The listing builds one solid part. Answer for the finished solid, in the listing's coordinates (mm). Give positions to 0.01 mm unless a question says otherwise; leave off trailing zeros. Write each loop counter-clockwise with the first axis right and the second up, starting at its lowest first coordinate (ties: lowest second). Pieces come first, ordered by that corner, then holes.
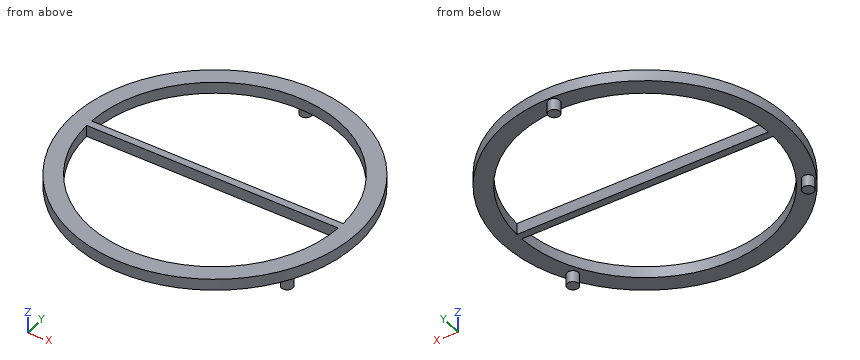
Autodesk Inventor part; units mm, degrees
ref_plane "YZ Plane" through (0, 0, 0) normal (1, 0, 0) x (0, 1, 0)
ref_plane "XZ Plane" through (0, 0, 0) normal (0, 1, 0) x (-1, 0, 0)
ref_plane "XY Plane" through (0, 0, 0) normal (0, 0, 1) x (1, 0, 0)
sketch "Sketch1" plane through (0, 0, 0) normal (0, 0, 1) x (1, 0, 0)
  circle A0 centre (0, 0) radius 250
  circle A1 centre (0, 0) radius 220
  dimension "d0" = 500
  dimension "d1" = 30
extrude "Extrusion1" add sketch "Sketch1" along normal blind 20
sketch "Sketch2" plane through (0, 0, 0) normal (0, 0, -1) x (-1, 0, 0)
  circle A0 centre (0, 237.6296) radius 10
  circle A1 centre (-205.7933, -118.8148) radius 10
  circle A2 centre (205.7933, -118.8148) radius 10
  point P0 (0, 0)
  dimension "d4" = 20
  dimension "d7" = 360
extrude "Extrusion2" add sketch "Sketch2" along normal blind 20
sketch "Sketch4" plane through (0, 0, 20) normal (0, 0, 1) x (1, 0, 0)
  line L0 (-238.2034, -6.414) -> (238.2034, -6.414)
  line L1 (238.2034, -6.414) -> (238.2034, 6.414)
  line L2 (238.2034, 6.414) -> (-238.2034, 6.414)
  line L3 (-238.2034, 6.414) -> (-238.2034, -6.414)
  line L4 (-238.2034, -6.414) -> (238.2034, 6.414) construction
  line L5 (238.2034, -6.414) -> (-238.2034, 6.414) construction
  point P0 (0, 0)
extrude "Extrusion3" add sketch "Sketch4" against normal blind 20
properties part number "platforma" material "Steel"
Item 1: A cutting plane is placed at A-A, the plane x = 0. Give the vertices of the cut face in (y, z).
Conclusion:
outline: (-250, 0) - (-220, 0) - (-220, 20) - (-250, 20) - close; (-6.41, 0) - (6.41, 0) - (6.41, 20) - (-6.41, 20) - close; (220, 0) - (227.63, 0) - (227.63, -20) - (247.63, -20) - (247.63, 0) - (250, 0) - (250, 20) - (220, 20) - close
Item 2: Consider probe 1 along Y at (x, z) = (32, 9.5); probe 2 along Y at (x, z) = (179, 8.5); probe 3 along X at (y, z) = (38.5, 16). Determine where each line is inside the solid, lowest interval first.
Conclusion:
probe 1: y = -247.94 to -217.66, -6.41 to 6.41, 217.66 to 247.94
probe 2: y = -174.53 to -127.9, -6.41 to 6.41, 127.9 to 174.53
probe 3: x = -247.02 to -216.61, 216.61 to 247.02
Item 3: A cutting plane is placed at C-C, the plane z = 13.5. Give the vertices of the cut face in (x, y), plus the area to 3 significant figures.
Conclusion:
outline: circle Ø500 at (0, 0); hole (-219.91, -6.41) arc R220 ccw to (219.91, -6.41) - close; hole (-219.91, 6.41) - (219.91, 6.41) arc R220 ccw to start
area: 49,900 mm2
Item 4: Each of these flat-tipped pins is pushed along its axis until it touches: P1, Ø4, axis at y = -42, z = 14.5, coming from the -X side; P2, Ø5, axis at x = 147.5, z = -3, coming from the +Y side; P3, Ø2, axis at x = 196.5, z = -12.5, coming from the -Y side. Where does it stop, or does it pass through?
Conclusion:
P1: stops at x = -246.78
P2: passes through
P3: stops at y = -124.4
Item 5: A cutting plane is placed at B-B, the plane y = 167. Give the vertices of the cut face in (x, z).
Conclusion:
outline: (-186.04, 0) - (-143.22, 0) - (-143.22, 20) - (-186.04, 20) - close; (143.22, 0) - (186.04, 0) - (186.04, 20) - (143.22, 20) - close
Item 6: A cutting plane is placed at D-D, the plane y = 0. Give the vertices of the cut face in (x, z), plus the area to 3 significant figures.
Conclusion:
outline: (-250, 0) - (250, 0) - (250, 20) - (-250, 20) - close
area: 10,000 mm2
